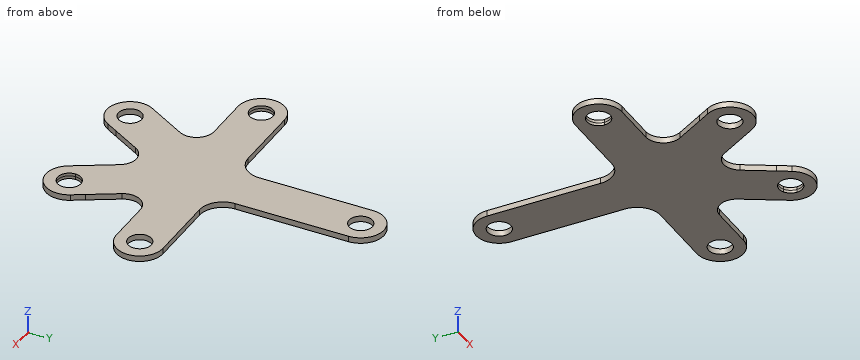
from build123d import *

# Parameters (mm, degrees)
F0_R     = 2
F1_DEPTH = 0.5


# Not quite as in the source:
# - a pattern or mirror of a feature is missing from the dataset's text; its kind, count and spacing are read off the source's solid


with BuildPart() as f1:
    # F0 (on Top) → F1 (new body)
    with BuildSketch(Plane.XY):
        with BuildLine():
            ThreePointArc((-20, 4), (-17.1715728753, 2.8284271247), (-16, 0))
            Line((-16, 0), (0, 0))
            Line((0, 0), (8, -13.8564064606))
            ThreePointArc((8, -13.8564064606), (10, -13.3205080757), (12, -13.8564064606))
            Line((12, -13.8564064606), (12.3094010768, -13.3205080757))
            Line((12.3094010768, -13.3205080757), (9.5262794416, -8.5))
            ThreePointArc((9.5262794416, -8.5), (9.5262794416, -5.5), (12.124355653, -4))
            Line((12.124355653, -4), (17.6905989232, -4))
            Line((17.6905989232, -4), (18, -3.4641016151))
            ThreePointArc((18, -3.4641016151), (16.1362966948, 1.0352761804), (20, 4))
            Line((20, 4), (8, 4))
            ThreePointArc((8, 4), (5.1715728753, 5.1715728753), (4, 8))
            Line((4, 8), (4, 27.5))
            ThreePointArc((4, 27.5), (0, 23.5), (-4, 27.5))
            Line((-4, 27.5), (-4, 8))
            ThreePointArc((-4, 8), (-5.1715728753, 5.1715728753), (-8, 4))
            Line((-8, 4), (-20, 4))
        make_face()
        with BuildLine():
            Line((0, 0), (-16, 0))
            ThreePointArc((-16, 0), (-16.5358983849, -2), (-18, -3.4641016151))
            Line((-18, -3.4641016151), (-17.6905989232, -4))
            Line((-17.6905989232, -4), (-12.124355653, -4))
            ThreePointArc((-12.124355653, -4), (-9.5262794416, -5.5), (-9.5262794416, -8.5))
            Line((-9.5262794416, -8.5), (-12.3094010768, -13.3205080757))
            Line((-12.3094010768, -13.3205080757), (-12, -13.8564064606))
            ThreePointArc((-12, -13.8564064606), (-10, -13.3205080757), (-8, -13.8564064606))
            Line((-8, -13.8564064606), (0, 0))
        make_face()
        with BuildLine():
            Line((8, -13.8564064606), (0, 0))
            Line((0, 0), (-8, -13.8564064606))
            ThreePointArc((-8, -13.8564064606), (-6.5358983849, -15.3205080757), (-6, -17.3205080757))
            Line((-6, -17.3205080757), (-5.3811978465, -17.3205080757))
            Line((-5.3811978465, -17.3205080757), (-2.5980762114, -12.5))
            ThreePointArc((-2.5980762114, -12.5), (0, -11), (2.5980762114, -12.5))
            Line((2.5980762114, -12.5), (5.3811978465, -17.3205080757))
            Line((5.3811978465, -17.3205080757), (6, -17.3205080757))
            ThreePointArc((6, -17.3205080757), (6.5358983849, -15.3205080757), (8, -13.8564064606))
        make_face()
        with BuildLine():
            Line((-9, -15.5884572681), (-8, -13.8564064606))
            ThreePointArc((-8, -13.8564064606), (-10, -13.3205080757), (-12, -13.8564064606))
            Line((-12, -13.8564064606), (-11, -15.5884572681))
            ThreePointArc((-11, -15.5884572681), (-10, -15.3205080757), (-9, -15.5884572681))
        make_face()
        with BuildLine():
            ThreePointArc((-6.5358983849, -19.3205080757), (-6.1362966948, -18.3557842561), (-6, -17.3205080757))
            Line((-6, -17.3205080757), (-8, -17.3205080757))
            ThreePointArc((-8, -17.3205080757), (-11, -19.0525588833), (-11, -15.5884572681))
            Line((-11, -15.5884572681), (-12, -13.8564064606))
            ThreePointArc((-12, -13.8564064606), (-12.8284271247, -14.4920809509), (-13.4641016151, -15.3205080757))
            ThreePointArc((-13.4641016151, -15.3205080757), (-12, -20.7846096908), (-6.5358983849, -19.3205080757))
        make_face()
        with BuildLine():
            ThreePointArc((-6, -17.3205080757), (-6.5358983849, -15.3205080757), (-8, -13.8564064606))
            Line((-8, -13.8564064606), (-9, -15.5884572681))
            ThreePointArc((-9, -15.5884572681), (-8.2679491924, -16.3205080757), (-8, -17.3205080757))
            Line((-8, -17.3205080757), (-6, -17.3205080757))
        make_face()
        with BuildLine():
            ThreePointArc((13.4641016151, -15.3205080757), (12.8284271247, -14.4920809509), (12, -13.8564064606))
            Line((12, -13.8564064606), (11, -15.5884572681))
            ThreePointArc((11, -15.5884572681), (11.7320508076, -16.3205080757), (12, -17.3205080757))
            ThreePointArc((12, -17.3205080757), (10, -19.3205080757), (8, -17.3205080757))
            Line((8, -17.3205080757), (6, -17.3205080757))
            ThreePointArc((6, -17.3205080757), (6.1362966948, -18.3557842561), (6.5358983849, -19.3205080757))
            ThreePointArc((6.5358983849, -19.3205080757), (11.0352761804, -21.1842113808), (14, -17.3205080757))
            ThreePointArc((14, -17.3205080757), (13.8637033052, -16.2852318953), (13.4641016151, -15.3205080757))
        make_face()
        with BuildLine():
            Line((9, -15.5884572681), (8, -13.8564064606))
            ThreePointArc((8, -13.8564064606), (6.5358983849, -15.3205080757), (6, -17.3205080757))
            Line((6, -17.3205080757), (8, -17.3205080757))
            ThreePointArc((8, -17.3205080757), (8.2679491924, -16.3205080757), (9, -15.5884572681))
        make_face()
        with BuildLine():
            ThreePointArc((12, -13.8564064606), (10, -13.3205080757), (8, -13.8564064606))
            Line((8, -13.8564064606), (9, -15.5884572681))
            ThreePointArc((9, -15.5884572681), (10, -15.3205080757), (11, -15.5884572681))
            Line((11, -15.5884572681), (12, -13.8564064606))
        make_face()
        with BuildLine():
            ThreePointArc((-19, -1.7320508076), (-21.7320508076, 1), (-18, 0))
            Line((-18, 0), (-16, 0))
            ThreePointArc((-16, 0), (-17.1715728753, 2.8284271247), (-20, 4))
            ThreePointArc((-20, 4), (-24, 0), (-20, -4))
            ThreePointArc((-20, -4), (-18.9647238196, -3.8637033052), (-18, -3.4641016151))
            Line((-18, -3.4641016151), (-19, -1.7320508076))
        make_face()
        with BuildLine():
            Line((-16, 0), (-18, 0))
            ThreePointArc((-18, 0), (-18.2679491924, -1), (-19, -1.7320508076))
            Line((-19, -1.7320508076), (-18, -3.4641016151))
            ThreePointArc((-18, -3.4641016151), (-16.5358983849, -2), (-16, 0))
        make_face()
        with BuildLine():
            ThreePointArc((20, 4), (16.1362966948, 1.0352761804), (18, -3.4641016151))
            ThreePointArc((18, -3.4641016151), (18.9647238196, -3.8637033052), (20, -4))
            ThreePointArc((20, -4), (22.8284271247, -2.8284271247), (24, 0))
            ThreePointArc((24, 0), (22.8284271247, 2.8284271247), (20, 4))
        make_face()
        with BuildLine():
            ThreePointArc((22, 0), (21, -1.7320508076), (19, -1.7320508076))
            ThreePointArc((19, -1.7320508076), (19, 1.7320508076), (22, 0))
        make_face(mode=Mode.SUBTRACT)
        with BuildLine():
            ThreePointArc((4, 27.5), (0, 31.5), (-4, 27.5))
            ThreePointArc((-4, 27.5), (0, 23.5), (4, 27.5))
        make_face()
        with Locations((0, 27.5)):
            Circle(F0_R, mode=Mode.SUBTRACT)
        with BuildLine():
            Line((-17.6905989232, -4), (-18, -3.4641016151))
            ThreePointArc((-18, -3.4641016151), (-18.9647238196, -3.8637033052), (-20, -4))
            Line((-20, -4), (-17.6905989232, -4))
        make_face()
        with BuildLine():
            Line((-12, -13.8564064606), (-12.3094010768, -13.3205080757))
            Line((-12.3094010768, -13.3205080757), (-13.4641016151, -15.3205080757))
            ThreePointArc((-13.4641016151, -15.3205080757), (-12.8284271247, -14.4920809509), (-12, -13.8564064606))
        make_face()
        with BuildLine():
            Line((-5.3811978465, -17.3205080757), (-6, -17.3205080757))
            ThreePointArc((-6, -17.3205080757), (-6.1362966948, -18.3557842561), (-6.5358983849, -19.3205080757))
            Line((-6.5358983849, -19.3205080757), (-5.3811978465, -17.3205080757))
        make_face()
        with BuildLine():
            ThreePointArc((6.5358983849, -19.3205080757), (6.1362966948, -18.3557842561), (6, -17.3205080757))
            Line((6, -17.3205080757), (5.3811978465, -17.3205080757))
            Line((5.3811978465, -17.3205080757), (6.5358983849, -19.3205080757))
        make_face()
        with BuildLine():
            Line((12.3094010768, -13.3205080757), (12, -13.8564064606))
            ThreePointArc((12, -13.8564064606), (12.8284271247, -14.4920809509), (13.4641016151, -15.3205080757))
            Line((13.4641016151, -15.3205080757), (12.3094010768, -13.3205080757))
        make_face()
        with BuildLine():
            Line((18, -3.4641016151), (17.6905989232, -4))
            Line((17.6905989232, -4), (20, -4))
            ThreePointArc((20, -4), (18.9647238196, -3.8637033052), (18, -3.4641016151))
        make_face()
    extrude(amount=F1_DEPTH)

    # F1_copies: F1 across plane


with BuildPart() as f1_1:
    add(f1.part)
    add(f1.part.mirror(Plane.XY.offset(0.5)))


solid = f1_1.part
Verification items for the finished model (mm, model axes). Give positions to 0.01 mm unless a question says otherwise; leave off trailing zeros. Write each loop counter-clockwise with the first axis right and the second up, starting at its lowest first coordinate (ties: lowest second). Pieces come first, ordered by that corner, then holes. Notation, with made-up numbers: M 56,82 L 88,82 A32 cw 88,119 Z; hole C 72,39.25 d6. An arc over 180 degrees is marked long. Put each result on its own line as item: value. Start each with the question number.
1. Section check B-B (z = 0.7). Record the cut outline in (x, y), and give its area (3 significant figures).
2. Section check A-A (x = 0). Record the cut outline in (y, z).
3. Section check C-C (y = 21.5). Record the cut outline in (x, z), and give its area (3 significant figures).
4. Go/stop test with a flat-tipped pin: pin 1 Ø0.5 at (x, z) = (16.5, 0.5) entering from +Y. Record where the tip stops, or that it passes through.
5. Scan lines: line 1 along X through (y, z) = (-15.5, 0.75); line 2 along Y through (x, z) = (-20, 0.3); line 3 along Y through (x, z) = (-10, 0.4). Record each from-to range of solid material in increasing order. Write a range as [from, to].
Answer list:
1. outline: M -20,-4 L -12.12,-4 A3 cw -9.53,-8.5 L -13.46,-15.32 A4 ccw -6.54,-19.32 L -2.6,-12.5 A3 cw 2.6,-12.5 L 6.54,-19.32 A4 ccw 13.46,-15.32 L 9.53,-8.5 A3 cw 12.12,-4 L 20,-4 A4 ccw 20,4 L 8,4 A4 cw 4,8 L 4,27.5 A4 ccw -4,27.5 L -4,8 A4 cw -8,4 L -20,4 A4 ccw Z; hole C -20,0 d4; hole C -10,-17.32 d4; hole C 0,27.5 d4; hole C 10,-17.32 d4; hole C 20,0 d4
1. area: 833 mm2
2. outline: M -11,0 L 25.5,0 L 25.5,1 L -11,1 Z; M 29.5,0 L 31.5,0 L 31.5,1 L 29.5,1 Z
3. outline: M -4,0 L 4,0 L 4,1 L -4,1 Z
3. area: 8.00 mm2
4. pin 1: y = 4
5. line 1: [-13.56, -10.83], [-9.17, -4.33], [4.33, 9.17], [10.83, 13.56]
5. line 2: [-4, -2], [2, 4]
5. line 3: [-21.32, -19.32], [-15.32, -9.32], [-4.88, 4]
